from build123d import *

# Parameters (mm, degrees)
SKETCH1_W           = 165
SKETCH1_H           = 75
BOSS_EXTRUDE1_DEPTH = 5
SKETCH3_R           = 4.5
SKETCH3_W           = 4
SKETCH3_H           = 5.5
BOSS_EXTRUDE3_DEPTH = 10
FILLET2_R           = 3
FILLET4_R           = 3
FILLET5_R           = 1
SKETCH4_R           = 4.5
CUT_EXTRUDE1_DEPTH  = 2


with BuildPart() as part:
    # Sketch1 → Boss-Extrude1 (new body)
    with BuildSketch(Plane(origin=(0, 0, 0), x_dir=(1, 0, 0), z_dir=(0, 1, 0))):
        Rectangle(SKETCH1_W, SKETCH1_H)
    extrude(amount=BOSS_EXTRUDE1_DEPTH)

    # Sketch3 → Boss-Extrude3 (add)
    with BuildSketch(Plane(origin=(0, 5, 0), x_dir=(1, 0, 0), z_dir=(0, 1, 0))):
        with Locations(Location((0, 0, 0), (0, 0, 270))):
            Circle(SKETCH3_R)
        with Locations((-71.25, 28.75)):
            Rectangle(SKETCH3_W, SKETCH3_H)
        with Locations((-71.25, -28.75)):
            Rectangle(SKETCH3_W, SKETCH3_H)
        with Locations((71.25, -28.75)):
            Rectangle(SKETCH3_W, SKETCH3_H)
        with Locations((71.25, 28.75)):
            Rectangle(SKETCH3_W, SKETCH3_H)
    extrude(amount=BOSS_EXTRUDE3_DEPTH)

    # Fillet2
    fillet2_edges = [part.edges().sort_by_distance(p)[0] for p in [
        (0, 5, -4.5),
    ]]
    fillet(fillet2_edges, radius=FILLET2_R)

    # Fillet4
    fillet4_edges = [part.edges().sort_by_distance(p)[0] for p in [
        (82.5, 2.5, 37.5),
        (-82.5, 2.5, 37.5),
        (-82.5, 2.5, -37.5),
        (82.5, 2.5, -37.5),
    ]]
    fillet(fillet4_edges, radius=FILLET4_R)

    # Fillet5
    fillet5_edges = [part.edges().sort_by_distance(p)[0] for p in [
        (-71.25, 5, -26),
        (-69.25, 5, -28.75),
        (-73.25, 5, -28.75),
        (-71.25, 5, -31.5),
        (73.25, 5, 28.75),
        (71.25, 5, 26),
        (71.25, 5, 31.5),
        (69.25, 5, 28.75),
        (73.25, 5, -28.75),
        (71.25, 5, -31.5),
        (71.25, 5, -26),
        (69.25, 5, -28.75),
        (-71.25, 5, 31.5),
        (-69.25, 5, 28.75),
        (-73.25, 5, 28.75),
        (-71.25, 5, 26),
    ]]
    fillet(fillet5_edges, radius=FILLET5_R)

    # Sketch4 → Cut-Extrude1 (cut)
    with BuildSketch(Plane.XZ):
        with Locations(Location((-22.5, -32.5, 0), (0, 0, 270))):
            Circle(SKETCH4_R)
        with Locations(Location((-22.5, 32.5, 0), (0, 0, 270))):
            Circle(SKETCH4_R)
        with Locations(Location((22.5, 32.5, 0), (0, 0, 90))):
            Circle(SKETCH4_R)
        with Locations(Location((22.5, -32.5, 0), (0, 0, 90))):
            Circle(SKETCH4_R)
    extrude(amount=-CUT_EXTRUDE1_DEPTH, mode=Mode.SUBTRACT)


solid = part.part
Could you check a few things on this model? Use its own coordinates, in mm. A direction names the side the tool comes from. Give positions to 0.01 mm unless a question says otherwise; leave off trailing zeros. Order: outer loops, then holes, each group sorted by start corner. A loop starts at its lowest first (then second) coordinate and runs counter-clockwise, first axis right, second up. Notation, with made-up numbers: (87.25, 4.25) -> (130.25, 4.25) arc R28 ccw to (130.25, 42.25) -> close; hole circle Ø6 at (-1.75, 39.25). An arc over 180 degrees is marked (long way). Return JSON: item names as keys, results as strings.
1. Imagine slicing it at C-C on z = 16.5. List the corners of the cut face in (x, y) for me, then the cut area to 3 significant figures.
Answer list:
{"outline": "(-82.5, 0) -> (82.5, 0) -> (82.5, 5) -> (-82.5, 5) -> close", "area": "825 mm2"}
2. I need wall thicknesses on line 1 (Z direction, x = 22.5, y = 0.8); line 2 (X direction, y = 0.65, z = 32.5); line 3 (Y direction, x = 45, z = 21). Which ranges of each line are inside material? Lowest first, please. Write a range as from..to.
Answer list:
{"line 1": "z = -37.5..-37, -28..28, 37..37.5", "line 2": "x = -82.5..-27, -18..18, 27..82.5", "line 3": "y = 0..5"}
3. On a 3-axis mill with a long thin cutter (end or side, diameter ignored), from which of +Z, -Z, +X, -X, +Y, -Y can I reach the whole of each face in a straight line? I mean faces 1 (the flat face through (73.25, 10, 29)), 2 (the flat face through (-22, 2, -32)), 3 (the flat face through (71, 10, 31.5)), 4 (the flat face through (-69.25, 10, 29)). Say none if no direction works.
Answer list:
{"face 1": "+Z, -Z, +X, +Y", "face 2": "-Y", "face 3": "+Z, +X, -X, +Y", "face 4": "+Z, -Z, +Y"}
4. Thinking about a two-plate mould opening in X: for faces 5 (the cylindrical face through (18.706, 0.986, 34.919)), 6 (the cylindrical face through (-18.706, 0.986, 30.081)), 7 (the cylindrical face through (-81.64, 2.54, -36.6)), 8 (the flat face through (71, 10, 26)), which applies, pulls with the +X half, pulls with the -X half, needs draft (parallel to the pull), parting line crosses it, or undercut?
Answer list:
{"face 5": "undercut", "face 6": "undercut", "face 7": "pulls with the -X half", "face 8": "needs draft"}
5. For pin 1 Ø2.5 at (x, z) = (-21, -32) entering from -Y; pin 2 Ø4.5 at (y, z) = (9, 28.5) entering from +X; pin 3 Ø5.5 at (x, z) = (22.5, 32.5) entering from +Y, each with a flat end and sliding along its axis, tell me the tip position at first contact or that it passes through.
Answer list:
{"pin 1": "stops at y = 2", "pin 2": "stops at x = 73.25", "pin 3": "stops at y = 5"}
6. Imagine slicing it at A-A on y = 12. List the corners of the cut face in (x, z) for me, then the cut area to 3 significant figures.
Answer list:
{"outline": "(-73.25, -31.5) -> (-69.25, -31.5) -> (-69.25, -26) -> (-73.25, -26) -> close; (-73.25, 26) -> (-69.25, 26) -> (-69.25, 31.5) -> (-73.25, 31.5) -> close; circle Ø9 at (0, 0); (69.25, -31.5) -> (73.25, -31.5) -> (73.25, -26) -> (69.25, -26) -> close; (69.25, 26) -> (73.25, 26) -> (73.25, 31.5) -> (69.25, 31.5) -> close", "area": "152 mm2"}
7. Imagine slicing it at D-D on x = 57.5. List the corners of the cut face in (y, z) for me, then the cut area to 3 significant figures.
Answer list:
{"outline": "(0, -37.5) -> (5, -37.5) -> (5, 37.5) -> (0, 37.5) -> close", "area": "375 mm2"}
8. Imagine slicing it at B-B on x = -22.5. List the corners of the cut face in (y, z) for me, then the cut area to 3 significant figures.
Answer list:
{"outline": "(0, -37.5) -> (5, -37.5) -> (5, 37.5) -> (0, 37.5) -> (0, 37) -> (2, 37) -> (2, 28) -> (0, 28) -> (0, -28) -> (2, -28) -> (2, -37) -> (0, -37) -> close", "area": "339 mm2"}
